For this review, take the finished solid that the model builds, in its own axes (mm). A direction names the side the tool comes from. Round coordinates to 2 decimals unless told otherwise and drop trailing zeros. Order: outer loops, then holes, each group sorted by start corner. A loop starts at its lowest first (then second) coordinate and runs counter-clockwise, first axis right, second up. Notation, with made-up numbers: (30, 59.5) -> (40, 59.5) arc R35 cw to (40, 95.5) -> close; hole circle Ø9 at (55.5, 73). An arc over 180 degrees is marked (long way). Answer in a Markdown table with one row per item.
```python
from build123d import *

# Parameters (mm, degrees)
BOSS_EXTRUDE1_DEPTH = 180
CUT_EXTRUDE1_DEPTH  = 176


with BuildPart() as part:
    # Sketch1 → Boss-Extrude1 (new body)
    with BuildSketch(Plane(origin=(0, 0, 0), x_dir=(1, 0, 0), z_dir=(0, 1, 0))):
        with BuildLine():
            Line((35, 0), (-35, 0))
            ThreePointArc((-35, 0), (-52.207293091, 5.425438671), (-63.190778624, 19.7393957))
            Line((-63.190778624, 19.7393957), (-81.908713693, 64.7393957))
            Line((-81.908713693, 64.7393957), (81.908713693, 64.7393957))
            Line((81.908713693, 64.7393957), (63.190778624, 19.7393957))
            ThreePointArc((63.190778624, 19.7393957), (52.207293091, 5.425438671), (35, 0))
        make_face()
    extrude(amount=BOSS_EXTRUDE1_DEPTH)

    # Sketch4 → Cut-Extrude1 (cut)
    with BuildSketch(Plane.XZ):
        with BuildLine():
            Line((-78.908713693, -64.7393957), (78.908713693, -64.7393957))
            Line((78.908713693, -64.7393957), (60.788869437, -21.764400459))
            add(Edge.make_bspline(
                [(35, -3), (54.769523096, -6.842262635), (60.788869437, -21.764400459)],
                knots=[0, 0, 0, 1, 1, 1], degree=2))
            Line((35, -3), (-35, -3))
            add(Edge.make_bspline(
                [(-35, -3), (-54.769523096, -6.842262635), (-60.788869437, -21.764400459)],
                knots=[0, 0, 0, 1, 1, 1], degree=2))
            Line((-60.788869437, -21.764400459), (-78.908713693, -64.7393957))
        make_face()
    extrude(amount=-CUT_EXTRUDE1_DEPTH, mode=Mode.SUBTRACT)


solid = part.part
```
Q1. Take a section at D-D, the plane x = 72.5. Write out the cut boundary in (y, z).
Answer key:
| item | result |
|---|---|
| outline | (0, -49.54) -> (176, -49.54) -> (176, -64.74) -> (180, -64.74) -> (180, -42.12) -> (0, -42.12) -> close |
Q2. Take a section at C-C, the plane z = -38.5. Write out the cut boundary in (x, y), then the cut area to 3 significant figures.
Answer key:
| item | result |
|---|---|
| outline | (-70.99, 0) -> (-67.85, 0) -> (-67.85, 176) -> (67.85, 176) -> (67.85, 0) -> (70.99, 0) -> (70.99, 180) -> (-70.99, 180) -> close |
| area | 1,680 mm^2 |
Q3. Take a section at A-A, the plane z = -29. Write out the cut boundary in (x, y).
Answer key:
| item | result |
|---|---|
| outline | (-67.04, 0) -> (-63.84, 0) -> (-63.84, 176) -> (63.84, 176) -> (63.84, 0) -> (67.04, 0) -> (67.04, 180) -> (-67.04, 180) -> close |
Q4. Tool access review of faces 1 (the face through (0, 89, 0)), 2 (the face through (-69.72, 86.77, -42.95)): name each direction out of +Z, -Z, +X, -X, +Y, -Y from which nothing blocks a thin tool from reaching the whole face with its end or side.
Answer key:
| item | result |
|---|---|
| face 1 | +Z, +X, -X, +Y, -Y |
| face 2 | -Z, -Y |
Q5. Clearance check with flat-ended pins moving along their axes: pin 1 Ø5 at (y, z) = (138.5, -47.5) entering from -X; pin 2 Ø4 at (x, y) = (42, 83) entering from -Z; pin 3 Ø1.5 at (x, y) = (22, 22) entering from -Z. State where each tip first meets the part, or that it passes through.
Answer key:
| item | result |
|---|---|
| pin 1 | stops at x = -75.78 |
| pin 2 | stops at z = -5.6 |
| pin 3 | stops at z = -3 |
Q6. Take a section at B-B, the plane x = 27. Write out the cut boundary in (y, z), then the cut area to 3 significant figures.
Answer key:
| item | result |
|---|---|
| outline | (0, -3) -> (176, -3) -> (176, -64.74) -> (180, -64.74) -> (180, 0) -> (0, 0) -> close |
| area | 787 mm^2 |
Q7. To check wall thickness, follow probe 1 along Y at (x, z) = (24.5, -54); probe 2 along Z at (x, y) = (21.5, 57); probe 3 along X at (y, z) = (101.5, -36). State the ranges of each line that lie inside material, in increasing order.
Answer key:
| item | result |
|---|---|
| probe 1 | y = 176 to 180 |
| probe 2 | z = -3 to 0 |
| probe 3 | x = -69.95 to -66.79, 66.79 to 69.95 |
